Work out the finished part from the listing and answer in its coordinate system (mm). Round coordinates to 2 decimals unless told otherwise and drop trailing zeros. Loops run counter-clockwise (first coordinate to the right, second up) from the corner with the lowest first, then second, coordinate; pieces in that order, holes last. Notation, with made-up numbers: (68.25, 84) - (104.25, 84) arc R31 ccw to (104.25, 111) - close; hole circle Ø6 at (72, 44.5). An arc over 180 degrees is marked (long way). Return JSON: item names as keys, results as strings.
from build123d import *

# Parameters (mm, degrees)
F1_DEPTH = 59.944
F2_R     = 41.967916
F3_DEPTH = 83.566


with BuildPart() as f1:
    # F0 (on Top) → F1 (new body)
    with BuildSketch(Plane.XY):
        Polygon((10.482761, -55.606968), (43.773731, -35.85922), (56.582486, 0.667455), (42.915667, 36.881821), (9.16813, 55.838773), (-28.869276, 48.668142), (-53.398427, 18.725147), (-52.941861, -19.979553), (-27.71321, -49.335598), align=None)
    extrude(amount=F1_DEPTH)

    # F2 (on Top) → F3 (cut)
    with BuildSketch(Plane.XY):
        Circle(F2_R)
    extrude(amount=F3_DEPTH, mode=Mode.SUBTRACT)


solid = f1.part
1) Section B-B (y = -18) is taken. Give the vertices of the cut face in (x, z), and give its area (3 significant figures).
Verdict:
{"outline": "(-52.97, 0) - (-37.91, 0) - (-37.91, 59.94) - (-52.97, 59.94) - close; (37.91, 0) - (50.04, 0) - (50.04, 59.94) - (37.91, 59.94) - close", "area": "1,630 mm2"}
2) Section C-C (x = 35.5) is taken. Give the vertices of the cut face in (y, z), and give its area (3 significant figures).
Verdict:
{"outline": "(-40.77, 0) - (-22.38, 0) - (-22.38, 59.94) - (-40.77, 59.94) - close; (22.38, 0) - (41.05, 0) - (41.05, 59.94) - (22.38, 59.94) - close", "area": "2,220 mm2"}
3) Flat-ended cylindrical pins translate along their axes: pin 1 (12 mm diameter, centred on y = 34.5, z = 33.5, fed in from -X); pin 2 (1.5 mm diameter, centred on x = -8, z = 30.5, fed in from -Y); pin 3 (8 mm diameter, centred on x = -34, z = 33.5, fed in from -Y). Find the tip coordinate at first contact, or state that the pin passes through.
Verdict:
{"pin 1": "stops at x = -45.39", "pin 2": "stops at y = -52.7", "pin 3": "stops at y = -46.67"}
4) Section A-A (z = 20) is taken. Give the vertices of the cut face in (x, y).
Verdict:
{"outline": "(-53.4, 18.73) - (-52.94, -19.98) - (-27.71, -49.34) - (10.48, -55.61) - (43.77, -35.86) - (56.58, 0.67) - (42.92, 36.88) - (9.17, 55.84) - (-28.87, 48.67) - close; hole circle Ø83.94 at (0, 0)"}
5) Determine the mould class of faces 1 (the flat face through (-11, -41, 0)), 2 (the cylindrical face through (-5.46, 41.61, 29.55)), 3 (the flat face through (-40.96, 33.91, 29.55)) for opening direction Y: pulls with the +Y half, pulls with the -Y half, needs draft (parallel to the pull), parting line crosses it, or undercut.
Verdict:
{"face 1": "needs draft", "face 2": "undercut", "face 3": "pulls with the +Y half"}
6) Find the intervals of material crossed by L1, parallel to Y at x = -22, z = 31.5; L2, parallel to Y at x = 9.5, z = 32; L3, parallel to X at y = 13.5, z = 37, in increasing order.
Verdict:
{"L1": "y = -50.27 to -35.74, 35.74 to 49.96", "L2": "y = -55.45 to -40.88, 40.88 to 55.65", "L3": "x = -53.34 to -39.74, 39.74 to 51.74"}
